For this review, take the finished solid that the model builds, in its own axes (mm). Face numbers are marked on the shaded views. A direction names the side the tool comes from. Round coordinates to 2 decimals unless told otherwise and drop trailing zeros. Loops run counter-clockwise (first coordinate to the right, second up) from the corner with the lowest first, then second, coordinate; pieces in that order, holes last.
1) Take a section at B-B (y = 1.9). State the section outline as (x, z) points, then the cut area to 3 significant figures.
2) Tool access review of the marked faces 1, 2, 3, 4 and 5: name each direction out of +Z, -Z, +X, -X, +Y, -Y from which nothing blocks a thin tool from reaching the whole face with its end or side.
3) Take a section at D-D (y = 0.45). State the section outline as (x, z) points.
4) Wall thickness on L1, parallel to Y at x = 8.5, z = -1.7; L2, parallel to X at y = 2.35, z = 0.6; L3, parallel to X at y = -0.35, z = -1.05: over which ranges is each line inside the solid? List them lowest first.
5) Insertion check: pin 1 (1 mm diameter, centred on y = 0, z = -1.5, fed in from +X). The pin has a flat end and moves straight along its axis. Give the tip position at first contact, or say it passes through.
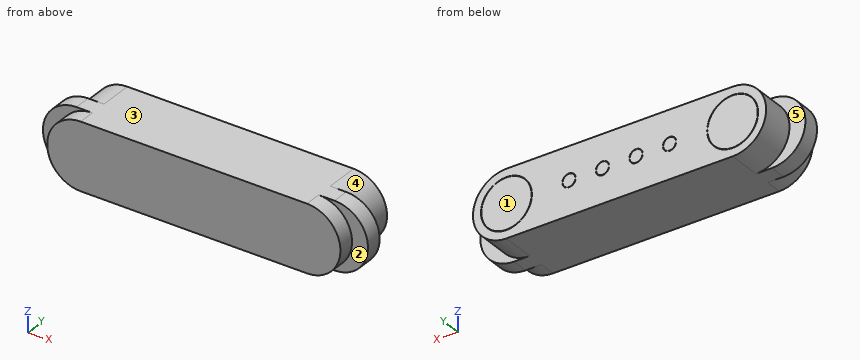
```python
from build123d import *

# Parameters (mm, degrees)
BOSS_EXTRUDE1_DEPTH = 2
BOSS_EXTRUDE2_START = -1
BOSS_EXTRUDE2_DEPTH = 0.5
SKETCH3_R           = 0.76
SKETCH3_R_2         = 0.75
SKETCH3_R_3         = 0.199685651
SKETCH3_R_4         = 0.189685651
CUT_EXTRUDE1_DEPTH  = 0.1
SCALE1_SCALE        = 2


with BuildPart() as part:
    # Sketch1 → Boss-Extrude1 (new body)
    with BuildSketch(Plane(origin=(0, 0, 0), x_dir=(1, 0, 0), z_dir=(0, 1, 0))):
        with BuildLine():
            Line((-3.375, 1), (3.375, 1))
            ThreePointArc((3.375, 1), (4.375, 0), (3.375, -1))
            Line((3.375, -1), (-3.375, -1))
            ThreePointArc((-3.375, -1), (-4.375, 0), (-3.375, 1))
        make_face()
    extrude(amount=BOSS_EXTRUDE1_DEPTH)

    # Sketch2 → Boss-Extrude2 (add)
    with BuildSketch(Plane(origin=(0, 2, 0), x_dir=(1, 0, 0), z_dir=(0, 1, 0)).offset(BOSS_EXTRUDE2_START)):
        with BuildLine():
            Line((-3.85, 1), (3.85, 1))
            ThreePointArc((3.85, 1), (4.85, 0), (3.85, -1))
            Line((3.85, -1), (-3.85, -1))
            ThreePointArc((-3.85, -1), (-4.85, 0), (-3.85, 1))
        make_face()
    extrude(amount=-BOSS_EXTRUDE2_DEPTH)

    # Sketch3 → Cut-Extrude1 (cut)
    with BuildSketch(Plane(origin=(0, 2, 0), x_dir=(1, 0, 0), z_dir=(0, 1, 0))):
        with Locations((-3.375, 0)):
            Circle(SKETCH3_R)
        with Locations((-3.375, 0)):
            Circle(SKETCH3_R_2, mode=Mode.SUBTRACT)
        with Locations((-1.492185541, -0.014395915)):
            Circle(SKETCH3_R_3)
        with Locations((-1.492185541, -0.014395915)):
            Circle(SKETCH3_R_4, mode=Mode.SUBTRACT)
        with Locations((-0.492185541, -0.014395915)):
            Circle(SKETCH3_R_3)
        with Locations((-0.492185541, -0.014395915)):
            Circle(SKETCH3_R_4, mode=Mode.SUBTRACT)
        with Locations((0.507814459, -0.014395915)):
            Circle(SKETCH3_R_3)
        with Locations((0.507814459, -0.014395915)):
            Circle(SKETCH3_R_4, mode=Mode.SUBTRACT)
        with Locations((1.507814459, -0.014395915)):
            Circle(SKETCH3_R_3)
        with Locations((1.507814459, -0.014395915)):
            Circle(SKETCH3_R_4, mode=Mode.SUBTRACT)
        with Locations((3.375, 0)):
            Circle(SKETCH3_R)
        with Locations((3.375, 0)):
            Circle(SKETCH3_R_2, mode=Mode.SUBTRACT)
    extrude(amount=-CUT_EXTRUDE1_DEPTH, mode=Mode.SUBTRACT)


with BuildPart() as part_1:
    # Scale1: scaled about (-1.117e-06, 0.99266013, -2.058e-06)
    add(part.part.scale(SCALE1_SCALE).moved(Location((1.117e-06, -0.99266013, 2.058e-06))))


solid = part_1.part
```
Response:
1. outline: (-6.75, -2) - (6.75, -2) arc R2 ccw to (6.75, 2) - (-6.75, 2) arc R2 ccw to start
1. area: 66.6 mm2
2. face 1: +Z, -Z, +X, -X, +Y
2. face 2: +X, -Y
2. face 3: +Z, +X, -X, +Y, -Y
2. face 4: +X, +Y
2. face 5: -X, +Y
3. outline: (-7.7, -2) - (7.7, -2) arc R2 ccw to (7.7, 2) - (-7.7, 2) arc R2 ccw to start
4. L1: y = 0.01 to 1.01
4. L2: x = -8.66 to 8.66
4. L3: x = -8.45 to 8.45
5. pin 1: stops at x = 9.43
